```python
from build123d import *

# Parameters (mm, degrees)
SKETCH1_W          = 50
SKETCH1_H          = 80
BASE_FLANGE1_DEPTH = 10
CUT_EXTRUDE1_REACH = 96.868
SKETCH6_R          = 2.5


# Sheet-metal steps are written as plain solids
with BuildPart() as part:
    # Sketch1 → Base-Flange1 (new body)
    with BuildSketch(Plane.XY):
        with Locations((25, 40)):
            Rectangle(SKETCH1_W, SKETCH1_H)
    extrude(amount=-BASE_FLANGE1_DEPTH)

    # Sketch6 → Cut-Extrude1 (cut, up to next)
    with BuildSketch(Plane.XY, mode=Mode.PRIVATE) as cut_extrude1_sk1:
        with Locations((40, 70)):
            Circle(SKETCH6_R)
    cut_extrude1_tool1 = extrude(cut_extrude1_sk1.sketch, amount=-CUT_EXTRUDE1_REACH, mode=Mode.PRIVATE) & part.part
    # Sketch6 → Cut-Extrude1 (cut, up to next)
    with BuildSketch(Plane.XY, mode=Mode.PRIVATE) as cut_extrude1_sk2:
        with Locations((10, 10)):
            Circle(SKETCH6_R)
    cut_extrude1_tool2 = extrude(cut_extrude1_sk2.sketch, amount=-CUT_EXTRUDE1_REACH, mode=Mode.PRIVATE) & part.part
    # Sketch6 → Cut-Extrude1 (cut, up to next)
    with BuildSketch(Plane.XY, mode=Mode.PRIVATE) as cut_extrude1_sk3:
        with Locations(Location((10, 70, 0), (0, 0, 180))):
            Circle(SKETCH6_R)
    cut_extrude1_tool3 = extrude(cut_extrude1_sk3.sketch, amount=-CUT_EXTRUDE1_REACH, mode=Mode.PRIVATE) & part.part
    # Sketch6 → Cut-Extrude1 (cut, up to next)
    with BuildSketch(Plane.XY, mode=Mode.PRIVATE) as cut_extrude1_sk4:
        with Locations(Location((40, 10, 0), (0, 0, 180))):
            Circle(SKETCH6_R)
    cut_extrude1_tool4 = extrude(cut_extrude1_sk4.sketch, amount=-CUT_EXTRUDE1_REACH, mode=Mode.PRIVATE) & part.part
    # Sketch6 → Cut-Extrude1 (cut, up to next)
    with BuildSketch(Plane.XY, mode=Mode.PRIVATE) as cut_extrude1_sk5:
        Polygon((40, 46.628826929), (40, 20), (10, 20), align=None)
    cut_extrude1_tool5 = extrude(cut_extrude1_sk5.sketch, amount=-CUT_EXTRUDE1_REACH, mode=Mode.PRIVATE) & part.part
    # Sketch6 → Cut-Extrude1 (cut, up to next)
    with BuildSketch(Plane.XY, mode=Mode.PRIVATE) as cut_extrude1_sk6:
        Polygon((40, 60), (10, 33.371173071), (10, 60), align=None)
    cut_extrude1_tool6 = extrude(cut_extrude1_sk6.sketch, amount=-CUT_EXTRUDE1_REACH, mode=Mode.PRIVATE) & part.part
    add(cut_extrude1_tool1.solids().sort_by_distance((40, 70, 0))[0], mode=Mode.SUBTRACT)
    add(cut_extrude1_tool2.solids().sort_by_distance((10, 10, 0))[0], mode=Mode.SUBTRACT)
    add(cut_extrude1_tool3.solids().sort_by_distance((10, 70, 0))[0], mode=Mode.SUBTRACT)
    add(cut_extrude1_tool4.solids().sort_by_distance((40, 10, 0))[0], mode=Mode.SUBTRACT)
    add(cut_extrude1_tool5.solids().sort_by_distance((30, 28.876276, 0))[0], mode=Mode.SUBTRACT)
    add(cut_extrude1_tool6.solids().sort_by_distance((20, 51.123724, 0))[0], mode=Mode.SUBTRACT)


solid = part.part
```
The model under review builds one solid part; all positions refer to its coordinate system, in mm. A direction names the side the tool comes from. Round coordinates to 2 decimals unless told otherwise and drop trailing zeros. Loops run counter-clockwise (first coordinate to the right, second up) from the corner with the lowest first, then second, coordinate; pieces in that order, holes last. Notation, with made-up numbers: M 11.25,3.25 L 46.25,3.25 A36 ccw 46.25,42.25 Z; hole C -31,-33 d1. An arc over 180 degrees is marked long. Put each result on its own line as item: value.
Q1. Consider section B-B, the plane z = -5.75. Give the boundary of the cut face in (x, y).
Result set:
outline: M 0,0 L 50,0 L 50,80 L 0,80 Z; hole C 10,10 d5; hole C 10,70 d5; hole M 10,20 L 40,20 L 40,46.63 Z; hole M 10,33.37 L 40,60 L 10,60 Z; hole C 40,10 d5; hole C 40,70 d5
Q2. For pin 1 (1.5 mm diameter, centred on x = 35, z = -9, fed in from -Y); pin 2 (4.5 mm diameter, centred on x = 10, y = 70, fed in from +Z), all flat-tipped, find the tip position at first contact; note any pin that passes through.
Result set:
pin 1: stops at y = 0
pin 2: passes through
Q3. Consider section D-D, the plane y = 24. Give the boundary of the cut face in (x, z), then the cut area to 3 significant figures.
Result set:
outline: M 0,-10 L 14.51,-10 L 14.51,0 L 0,0 Z; M 40,-10 L 50,-10 L 50,0 L 40,0 Z
area: 245 mm²
Q4. Machinability: for faces 5 (the flat face through (25.21, 46.87, -4.93)), 6 (the flat face through (25, 41, -10)), which of the approach directions +Z, -Z, +X, -X, +Y, -Y give a long, thin tool a straight path to every point of the face, cutting with its end or side? Answer none if there is none.
Result set:
face 5: +Z, -Z
face 6: -Z, +X, -X, +Y, -Y
Q5. Mouldability with a two-part tool opening along Y and no side actions: class faces 1 (the flat face through (40, 34, -5)), 2 (the flat face through (50, 39, -5)), 3 (the flat face through (25, 0, -5)), 4 (the flat face through (25, 80, -5)) as released by +Y, released by -Y, zero draft, split by the parting line, or undercut.
Result set:
face 1: undercut
face 2: zero draft
face 3: released by -Y
face 4: released by +Y
Q6. Consider section C-C, the plane y = 43. Give the boundary of the cut face in (x, z), then the cut area to 3 significant figures.
Result set:
outline: M 0,-10 L 10,-10 L 10,0 L 0,0 Z; M 20.85,-10 L 35.91,-10 L 35.91,0 L 20.85,0 Z; M 40,-10 L 50,-10 L 50,0 L 40,0 Z
area: 351 mm²
Q7. To check wall thickness, follow L1, parallel to Y at x = 29, z = -8; L2, parallel to X at y = 34.5, z = -1.75; L3, parallel to Y at x = 21.5, z = -4.75. State the ranges of each line that lie inside material, in increasing order.
Result set:
L1: y = 0 to 20, 36.86 to 50.24, 60 to 80
L2: x = 0 to 10, 11.27 to 26.34, 40 to 50
L3: y = 0 to 20, 30.21 to 43.58, 60 to 80
Q8. Consider section A-A, the plane x = 41. Give the boundary of the cut face in (y, z), then the cut area to 3 significant figures.
Result set:
outline: M 0,-10 L 7.71,-10 L 7.71,0 L 0,0 Z; M 12.29,-10 L 67.71,-10 L 67.71,0 L 12.29,0 Z; M 72.29,-10 L 80,-10 L 80,0 L 72.29,0 Z
area: 708 mm²
